Check sheet for the drawn part. Datum: minimum x, y, z corner. Units: mm. Coordinates: 2 decimals unless noted, no trailing zeros. Order: outer loops, then holes, each group sorted by start corner. A loop starts at its lowest first (then second) coordinate and runs counter-clockwise, first axis right, second up. Notation, with made-up numbers: (20, 55.25) - (46, 55.25) arc R19 cw to (46, 81.25) - close; hole circle Ø7 at (31.5, 65). An arc over 180 degrees is marked (long way). Put each result on its own line as item: value.
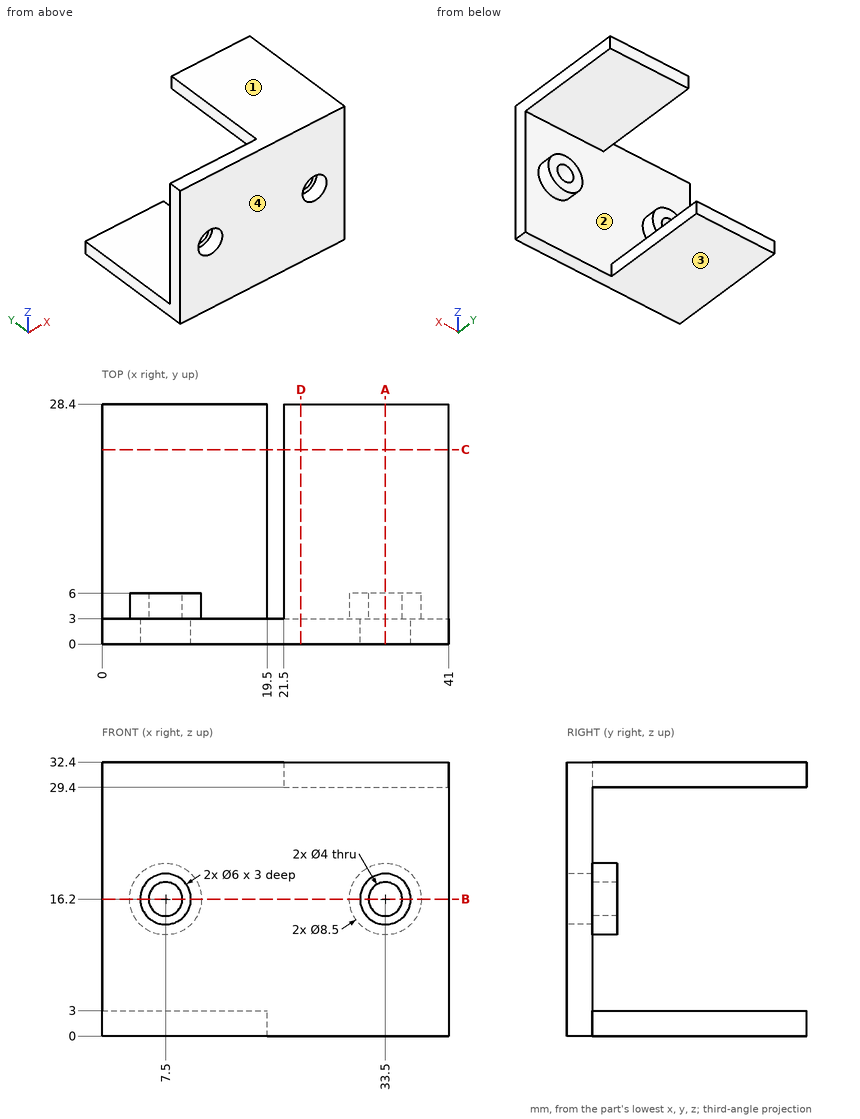
Q1. Section check A-A on x = 33.5. Record the boundary of the cut face in (y, z), then the cut area to 3 significant figures.
Answer block:
outline: (0, 0) - (3, 0) - (3, 11.95) - (6, 11.95) - (6, 14.2) - (3, 14.2) - (3, 13.2) - (0, 13.2) - close; (0, 19.2) - (3, 19.2) - (3, 18.2) - (6, 18.2) - (6, 20.45) - (3, 20.45) - (3, 29.4) - (28.4, 29.4) - (28.4, 32.4) - (0, 32.4) - close
area: 169 mm^2
Q2. Depth check by flat-ended pin: pin 1 Ø15.5 at (x, y) = (34.5, 22) entering from -Z; pin 2 Ø6 at (x, y) = (14.5, 23.5) entering from +Z; pin 3 Ø2 at (y, z) = (22.5, 4.5) entering from +X; pin 4 Ø15.5 at (x, y) = (11, 11) entering from +Z. Enter the tip coordinate at first touch or a pass-through.
Answer block:
pin 1: stops at z = 29.4
pin 2: stops at z = 3
pin 3: passes through
pin 4: stops at z = 20.45
Q3. Section check B-B on z = 16.2. Record the boundary of the cut face in (x, y).
Answer block:
outline: (0, 0) - (4.5, 0) - (4.5, 3) - (5.5, 3) - (5.5, 6) - (3.25, 6) - (3.25, 3) - (0, 3) - close; (9.5, 3) - (10.5, 3) - (10.5, 0) - (30.5, 0) - (30.5, 3) - (31.5, 3) - (31.5, 6) - (29.25, 6) - (29.25, 3) - (11.75, 3) - (11.75, 6) - (9.5, 6) - close; (35.5, 3) - (36.5, 3) - (36.5, 0) - (41, 0) - (41, 3) - (37.75, 3) - (37.75, 6) - (35.5, 6) - close
Q4. Section check C-C on y = 23. Record the boundary of the cut face in (x, z), then the cut area to 3 significant figures.
Answer block:
outline: (0, 0) - (19.5, 0) - (19.5, 3) - (0, 3) - close; (21.5, 29.4) - (41, 29.4) - (41, 32.4) - (21.5, 32.4) - close
area: 117 mm^2
Q5. Thickness scan on L1, parallel to Z at x = 7.5, y = 4.45; L2, parallel to Z at x = 7.5, y = 1.45; L3, parallel to Z at x = 19, y = 13. Record the ranges inside material, lowest first. Write a range as [from, to].
Answer block:
L1: z = [0, 3], [11.95, 14.2], [18.2, 20.45]
L2: z = [0, 13.2], [19.2, 32.4]
L3: z = [0, 3]
Q6. Draft check along Z on the marked faces 1, 2, 3 and 4. Enter one of: pulls with the +Z half, pulls with the -Z half, needs draft (parallel to the pull), parting line crosses it, or undercut.
Answer block:
face 1: pulls with the +Z half
face 2: undercut
face 3: pulls with the -Z half
face 4: needs draft
Q7. Section check D-D on x = 23.5. Record the boundary of the cut face in (y, z).
Answer block:
outline: (0, 0) - (3, 0) - (3, 29.4) - (28.4, 29.4) - (28.4, 32.4) - (0, 32.4) - close
